Check sheet for the modelled part. Datum: model origin and axes. Units: mm. Round coordinates to 2 decimals unless told otherwise and drop trailing zeros. Write each loop counter-clockwise with the first axis right and the second up, starting at its lowest first coordinate (ties: lowest second). Pieces come first, ordered by that corner, then holes.
Item 1: Section check C-C, the plane z = 22.5. Record the cut outline in (x, y).
Item 2: Material ranges on line 1 along X through (y, z) = (133.5, -31); line 2 along Z through (x, y) = (3.25, -33.5) (3 decimals); line 3 along Y through (x, z) = (7.75, 31), recorded low to high.
Item 3: Section check B-B, the plane y = 73.5. Record the cut outline in (x, z) (3 decimals).
Item 4: Section check A-A, the plane z = -32.5. Record the cut outline in (x, y), plus the area to 3 significant figures.
Item 5: Depth check by flat-ended pin: pin 1 (5 mm diameter, centred on x = -1.5, y = -226.5, fed in from +Z) (3 decimals); pin 2 (3 mm diameter, centred on x = -1.5, y = -120.5, fed in from -Z) (3 decimals). Enter the tip coordinate at first touch or a pass-through.
from build123d import *

# Parameters (mm, degrees)
F0_W     = 431.8
F0_H     = 76.2
F1_DEPTH = 10.31875
F2_W     = 9.525
F2_H     = 57.15
F3_DEPTH = 25.4
F4_W     = 9.525
F4_H     = 57.15
F5_DEPTH = 25.4
F6_W     = 7.9375
F6_H     = 431.8
F7_DEPTH = 9.525


with BuildPart() as f1:
    # F0 (on Right) → F1 (new body, symmetric)
    with BuildSketch(Plane.YZ):
        Rectangle(F0_W, F0_H)
    extrude(amount=F1_DEPTH, both=True)

    # F2 (on face) → F3 (join)
    with BuildSketch(Plane.XZ.offset(215.9)):
        Rectangle(F2_W, F2_H)
    extrude(amount=F3_DEPTH)

    # F4 (on face) → F5 (join)
    with BuildSketch(Plane(origin=(0, 215.9, 0), x_dir=(-1, 0, 0), z_dir=(0, 1, 0))):
        Rectangle(F4_W, F4_H)
    extrude(amount=F5_DEPTH)

    # F6 (on face) → F7 (cut)
    with BuildSketch(Plane(origin=(0, 0, -38.1), x_dir=(1, 0, 0), z_dir=(0, 0, -1))):
        Rectangle(F6_W, F6_H)
    extrude(amount=-F7_DEPTH, mode=Mode.SUBTRACT)


solid = f1.part
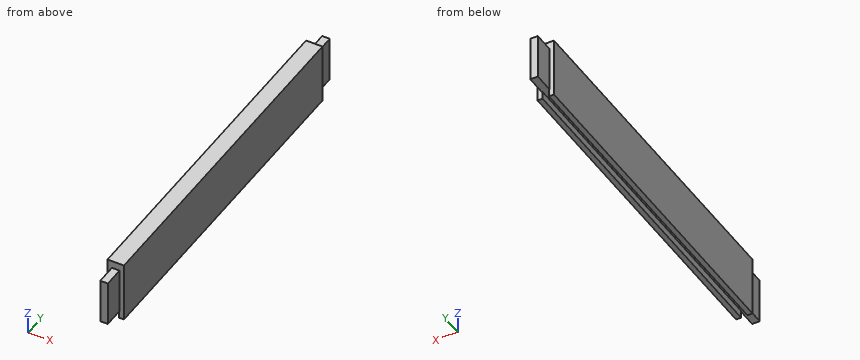
Values found:
1. outline: (-10.32, -215.9) - (-4.76, -215.9) - (-4.76, -241.3) - (4.76, -241.3) - (4.76, -215.9) - (10.32, -215.9) - (10.32, 215.9) - (4.76, 215.9) - (4.76, 241.3) - (-4.76, 241.3) - (-4.76, 215.9) - (-10.32, 215.9) - close
2. line 1: x = -10.32 to -3.97, 3.97 to 10.32
2. line 2: z = -28.575 to 38.1
2. line 3: y = -215.9 to 215.9
3. outline: (-10.319, -38.1) - (-3.969, -38.1) - (-3.969, -28.575) - (3.969, -28.575) - (3.969, -38.1) - (10.319, -38.1) - (10.319, 38.1) - (-10.319, 38.1) - close
4. outline: (-10.32, -215.9) - (-3.97, -215.9) - (-3.97, 215.9) - (-10.32, 215.9) - close; (3.97, -215.9) - (10.32, -215.9) - (10.32, 215.9) - (3.97, 215.9) - close
4. area: 5,480 mm2
5. pin 1: stops at z = 28.575
5. pin 2: stops at z = -28.575
